Build history of the part. All positions in model axes, mm. A direction names the side the tool comes from. Give positions to 0.01 mm unless a question says otherwise; leave off trailing zeros. Loops run counter-clockwise (first coordinate to the right, second up) from the corner with the lowest first, then second, coordinate; pieces in that order, holes last. Notation, with made-up numbers: (32, -9.75) - (71, -9.75) arc R29 cw to (71, 10.25) - close; hole circle Ø6 at (70.25, 72). An arc over 180 degrees is marked (long way). Return JSON: item names as keys, results as strings. Group by question number.
1) Slice it at C-C (y = 35). List the corners of the cut face in (x, z).
2) Slice it at B-B (x = 0). List the corners of the cut face in (y, z).
3) Drop flat-ended pins along their axis: pin 1 (6.5 mm diameter, centred on y = 11.5, z = -5, fed in from -X); pin 2 (9.5 mm diameter, centred on x = -31, z = 0, fed in from +Y); pin 3 (4 mm diameter, centred on y = 12.5, z = 1, fed in from +X); pin 4 (3.5 mm diameter, centred on x = 0, z = 0, fed in from -Y). Give the stop position or say it passes through.
4) Slice it at A-A (y = 14.5). List the corners of the cut face in (x, z).
5) 3-axis set-ups, long thin cutter, end or side, ignore diameter. For faces 1 (the face through (-38, 19, 0)), 2 (the face through (-22.5, 29, 0.1)), 3 (the face through (22, 12, 0)): which of +Z, -Z, +X, -X, +Y, -Y reach the whole face in a straight line?
6) Slice it at D-D (x = -31). List the corners of the cut face in (y, z), and give its area (3 significant figures).
7) Mould opens along X. For faces 4 (the face through (-2.11, 31.59, -1.34)), 5 (the face through (-1, 22, 18)), 6 (the face through (-48, 24, 0)), 7 (the face through (0, 38, 4)) say: released by +X, released by -X, zero draft, split by the parting line, or undercut.
8) Drill centre lines: probe 1 along Z at (x, y) = (0, 23); probe 2 along Z at (x, y) = (0, 35); probe 3 along Y at (x, z) = (-37, 1). Where is each one in solid material? Low to high. Write a range as from..to.
```python
from build123d import *

# Parameters (mm, degrees)
BOSS_EXTRUDE1_DEPTH            = 18
CUT_EXTRUDE1_REACH             = 24
SKETCH2_R                      = 4.221723053
CUT_EXTRUDE1_DIRECTION_2_DEPTH = 11
SKETCH3_R                      = 8.5
CUT_EXTRUDE2_DEPTH             = 36
SKETCH18_W                     = 2.5
SKETCH18_H                     = 13
M5_TAPPED_HOLE1_D              = 4.2


with BuildPart() as part:
    # Sketch1 → Boss-Extrude1 (new body, symmetric)
    with BuildSketch(Plane.XY):
        with BuildLine():
            Line((18.027756377, 6), (22, 6))
            Line((22, 6), (22, 19))
            Line((22, 19), (49, 19))
            Line((49, 19), (49, 28))
            Line((49, 28), (25.690465157, 28))
            ThreePointArc((25.690465157, 28), (0, 38), (-25.690465157, 28))
            Line((-25.690465157, 28), (-49, 28))
            Line((-49, 28), (-49, 19))
            Line((-49, 19), (-22, 19))
            Line((-22, 19), (-22, 6))
            Line((-22, 6), (-18.027756377, 6))
            ThreePointArc((-18.027756377, 6), (0, 19), (18.027756377, 6))
        make_face()
    extrude(amount=BOSS_EXTRUDE1_DEPTH, both=True)

    # Sketch2 → Cut-Extrude1 (cut, up to next)
    with BuildSketch(Plane(origin=(0, 28, 0), x_dir=(1, 0, 0), z_dir=(0, 1, 0)), mode=Mode.PRIVATE) as cut_extrude1_sk1:
        with Locations((-31, 0)):
            Circle(SKETCH2_R)
    cut_extrude1_tool1 = extrude(cut_extrude1_sk1.sketch, amount=-CUT_EXTRUDE1_REACH, mode=Mode.PRIVATE) & part.part
    add(cut_extrude1_tool1.solids().sort_by_distance((-31, 28, 0))[0], mode=Mode.SUBTRACT)
    # Sketch2 → Cut-Extrude1 (cut, up to next)
    with BuildSketch(Plane(origin=(0, 28, 0), x_dir=(1, 0, 0), z_dir=(0, 1, 0)), mode=Mode.PRIVATE) as cut_extrude1_sk2:
        with Locations((31, 0)):
            Circle(SKETCH2_R)
    cut_extrude1_tool2 = extrude(cut_extrude1_sk2.sketch, amount=-CUT_EXTRUDE1_REACH, mode=Mode.PRIVATE) & part.part
    add(cut_extrude1_tool2.solids().sort_by_distance((31, 28, 0))[0], mode=Mode.SUBTRACT)
    # Sketch2 → Cut-Extrude1 (cut, up to next)
    with BuildSketch(Plane(origin=(0, 28, 0), x_dir=(1, 0, 0), z_dir=(0, 1, 0)), mode=Mode.PRIVATE) as cut_extrude1_sk3:
        with BuildLine():
            Line((-44.497190923, 18), (-49, 18))
            Line((-49, 18), (-49, -18))
            Line((-49, -18), (-44.497190923, -18))
            ThreePointArc((-44.497190923, -18), (-48, 0), (-44.497190923, 18))
        make_face()
    cut_extrude1_tool3 = extrude(cut_extrude1_sk3.sketch, amount=-CUT_EXTRUDE1_REACH, mode=Mode.PRIVATE) & part.part
    add(cut_extrude1_tool3.solids().sort_by_distance((-48.362805, 28, 0))[0], mode=Mode.SUBTRACT)
    # Sketch2 → Cut-Extrude1 (cut, up to next)
    with BuildSketch(Plane(origin=(0, 28, 0), x_dir=(1, 0, 0), z_dir=(0, 1, 0)), mode=Mode.PRIVATE) as cut_extrude1_sk4:
        with BuildLine():
            Line((44.497190923, -18), (49, -18))
            Line((49, -18), (49, 18))
            Line((49, 18), (44.497190923, 18))
            ThreePointArc((44.497190923, 18), (48, 0), (44.497190923, -18))
        make_face()
    cut_extrude1_tool4 = extrude(cut_extrude1_sk4.sketch, amount=-CUT_EXTRUDE1_REACH, mode=Mode.PRIVATE) & part.part
    add(cut_extrude1_tool4.solids().sort_by_distance((46.748595, 28, 17.637195))[0], mode=Mode.SUBTRACT)

    # Sketch2 → Cut-Extrude1 direction 2 (cut)
    with BuildSketch(Plane(origin=(0, 28, 0), x_dir=(1, 0, 0), z_dir=(0, 1, 0))):
        with Locations((-31, 0)):
            Circle(SKETCH2_R)
        with Locations((31, 0)):
            Circle(SKETCH2_R)
        with BuildLine():
            Line((-44.497190923, 18), (-49, 18))
            Line((-49, 18), (-49, -18))
            Line((-49, -18), (-44.497190923, -18))
            ThreePointArc((-44.497190923, -18), (-48, 0), (-44.497190923, 18))
        make_face()
        with BuildLine():
            Line((44.497190923, -18), (49, -18))
            Line((49, -18), (49, 18))
            Line((49, 18), (44.497190923, 18))
            ThreePointArc((44.497190923, 18), (48, 0), (44.497190923, -18))
        make_face()
    extrude(amount=CUT_EXTRUDE1_DIRECTION_2_DEPTH, mode=Mode.SUBTRACT)

    # Sketch3 → Cut-Extrude2 (cut)
    with BuildSketch(Plane(origin=(0, 28, 0), x_dir=(1, 0, 0), z_dir=(0, 1, 0))):
        with Locations((-31, 0)):
            Circle(SKETCH3_R)
        with Locations((31, 0)):
            Circle(SKETCH3_R)
    extrude(amount=CUT_EXTRUDE2_DEPTH, mode=Mode.SUBTRACT)

    # Sketch18 → M6 Tapped Hole2 (revolve, cut)
    with BuildSketch(Plane(origin=(0, 25, 0), x_dir=(0, 0, -1), z_dir=(1, 0, 0))):
        with Locations((1.25, 6.5)):
            Rectangle(SKETCH18_W, SKETCH18_H)
    revolve(axis=Axis((0, 18.65, 0), (0, 1, 0)), mode=Mode.SUBTRACT)

    # M5 Tapped Hole1 (through all)
    with Locations(Plane(origin=(0, 25, 0), x_dir=(1, 0, 0), z_dir=(0, 1, 0))):
        with Locations((0, 0)):
            Hole(M5_TAPPED_HOLE1_D / 2)


solid = part.part
```
Results:
{
 "1": {"outline": "(-14.8, -18) - (14.8, -18) - (14.8, 18) - (-14.8, 18) - close; hole circle Ø5 at (0, 0)"},
 "2": {"outline": "(19, -18) - (38, -18) - (38, -2.5) - (25, -2.5) - (25, -2.1) - (19, -2.1) - close; (19, 2.1) - (25, 2.1) - (25, 2.5) - (38, 2.5) - (38, 18) - (19, 18) - close"},
 "3": {"pin 1": "x = -22", "pin 2": "y = 28", "pin 3": "x = 22", "pin 4": "through"},
 "4": {"outline": "(-22, -18) - (-12.28, -18) - (-12.28, 18) - (-22, 18) - close; (12.28, -18) - (22, -18) - (22, 18) - (12.28, 18) - close"},
 "5": {"face 1": "+Z, -Z, -X, -Y", "face 2": "-X, +Y", "face 3": "+Z, -Z, +X, -Y"},
 "6": {"outline": "(19, -18) - (28, -18) - (28, -4.22) - (19, -4.22) - close; (19, 4.22) - (28, 4.22) - (28, 18) - (19, 18) - close", "area": "248 mm2"},
 "7": {"face 4": "undercut", "face 5": "zero draft", "face 6": "released by -X", "face 7": "split by the parting line"},
 "8": {"probe 1": "-18..-2.1, 2.1..18", "probe 2": "-18..-2.5, 2.5..18", "probe 3": "19..28"}
}
